Verification items for the finished model (mm, model axes). A direction names the side the tool comes from. Round coordinates to 2 decimals unless told otherwise and drop trailing zeros. Loops run counter-clockwise (first coordinate to the right, second up) from the corner with the lowest first, then second, coordinate; pieces in that order, holes last. Notation, with made-up numbers: M 25,11.5 L 79,11.5 A13 cw 79,19.5 Z; hole C -2.75,68.25 d3. An arc over 180 degrees is marked long. Answer as CSV lines item,"result".
```python
from build123d import *

# Parameters (mm, degrees)
ESQUISSE1_W             = 28
ESQUISSE1_H             = 40
ESQUISSE1_R             = 1.5
BOSS_EXTRU_1_DEPTH      = 1.5
ESQUISSE3_R             = 1.5
ESQUISSE3_W             = 3
ESQUISSE3_H             = 22
BOSS_EXTRU_2_DEPTH      = 1.5
CONG_1_R                = 6
ESQUISSE4_R             = 1.5
ESQUISSE4_W             = 6
ESQUISSE4_H             = 18
ENL_V_MAT_EXTRU_1_DEPTH = 36.387144698
CONG_2_R                = 2


with BuildPart() as part:
    # Esquisse1 → Boss.-Extru.1 (new body)
    with BuildSketch(Plane.XY):
        Rectangle(ESQUISSE1_W, ESQUISSE1_H)
        with Locations((-7.5, 8)):
            Circle(ESQUISSE1_R, mode=Mode.SUBTRACT)
        with Locations(Location((7.5, 8, 0), (0, 0, 180))):
            Circle(ESQUISSE1_R, mode=Mode.SUBTRACT)
        with Locations((7.5, -8)):
            Circle(ESQUISSE1_R, mode=Mode.SUBTRACT)
        with Locations(Location((-7.5, -8, 0), (0, 0, 180))):
            Circle(ESQUISSE1_R, mode=Mode.SUBTRACT)
    extrude(amount=BOSS_EXTRU_1_DEPTH)

    # Esquisse3 → Boss.-Extru.2 (add)
    # profile 1 of 2: a face of its own
    with BuildSketch(Plane.XY.offset(1.5)):
        with BuildLine():
            Line((2, 20), (2, 25))
            ThreePointArc((2, 25), (8, 31), (14, 25))
            Line((14, 25), (14, 20))
            ThreePointArc((14, 20), (8, 14), (2, 20))
        make_face()
        with Locations((8, 25)):
            Circle(ESQUISSE3_R, mode=Mode.SUBTRACT)
    # profile 2 of 2: a face of its own
    with BuildSketch(Plane.XY.offset(1.5)):
        with Locations((-15.5, -9)):
            Rectangle(ESQUISSE3_W, ESQUISSE3_H)
    extrude(amount=-BOSS_EXTRU_2_DEPTH)

    # Congé1
    cong_1_edges = [part.edges().sort_by_distance(p)[0] for p in [
        (2, 20, 0.75),
    ]]
    fillet(cong_1_edges, radius=CONG_1_R)

    # Esquisse4 → Enlèv. mat.-Extru.1 (cut, through all)
    with BuildSketch(Plane.XY.offset(1.5)):
        with Locations((-13.7, -3)):
            Circle(ESQUISSE4_R)
        with Locations(Location((-13.7, -15, 0), (0, 0, 180))):
            Circle(ESQUISSE4_R)
        with Locations((-14, 11)):
            Rectangle(ESQUISSE4_W, ESQUISSE4_H)
    extrude(amount=-ENL_V_MAT_EXTRU_1_DEPTH, mode=Mode.SUBTRACT)

    # Congé2
    cong_2_edges = [part.edges().sort_by_distance(p)[0] for p in [
        (-17, 2, 0.75),
        (-17, -20, 0.75),
        (14, -20, 0.75),
        (-11, 2, 0.75),
        (-11, 20, 0.75),
    ]]
    fillet(cong_2_edges, radius=CONG_2_R)


solid = part.part
```
1) Draft check along Y on faces 3 (the cylindrical face through (13.4, -19.43, 0.76)), 4 (the cylindrical face through (-12.27, -2.55, 0.76)), 5 (the flat face through (2, 0, 1.5)). Enter one of: +Y half, -Y half, draft (parallel to the pull), parting line (faces both ways), or undercut.
Here are the results:
face 3,"-Y half"
face 4,"undercut"
face 5,"draft"
2) Material ranges on probe 1 along Y at (x, z) = (-13.7, 0.6); probe 2 along Y at (x, z) = (8, 0.8); probe 3 along Y at (x, z) = (7.5, 0.45), recorded low to high.
Here are the results:
probe 1,"y = -20 to -16.5, -13.5 to -4.5, -1.5 to 2"
probe 2,"y = -20 to -9.41, -6.59 to 6.59, 9.41 to 23.5, 26.5 to 31"
probe 3,"y = -20 to -9.5, -6.5 to 6.5, 9.5 to 23.59, 26.41 to 30.98"
3) Section check C-C (y = -15). Record the cut outline in (x, z).
Here are the results:
outline,"M -17,0 L -15.2,0 L -15.2,1.5 L -17,1.5 Z; M -12.2,0 L 14,0 L 14,1.5 L -12.2,1.5 Z"
4) Section check A-A (y = 8). Record the cut outline in (x, z).
Here are the results:
outline,"M -11,0 L -9,0 L -9,1.5 L -11,1.5 Z; M -6,0 L 6,0 L 6,1.5 L -6,1.5 Z; M 9,0 L 14,0 L 14,1.5 L 9,1.5 Z"
5) Section check D-D (z = 0.7). State how many separate pieces and enclosed holes the cut face has, plus the area to 3 significant figures.
Here are the results:
separate pieces,"1"
enclosed holes,"7"
area,"1,200 mm^2"
6) Go/stop test with a flat-tipped pin: pin 1 (2.5 mm diameter, centred on x = 7.5, y = -8, fed in from -Z). Record where the tip stops, or that it passes through.
Here are the results:
pin 1,"passes through"
7) Set-up check for faces 1 (the flat face through (-14, 2, 1)), 2 (the cylindrical face through (-16.43, -19.4, 0.74)): record each of +Z, -Z, +X, -X, +Y, -Y from which the full face is reachable in a straight line by a thin tool's end or side.
Here are the results:
face 1,"+Z, -Z, -X, +Y"
face 2,"+Z, -Z, -X, -Y"
8) Section check B-B (x = -7.5). Record the cut outline in (y, z).
Here are the results:
outline,"M -20,0 L -9.5,0 L -9.5,1.5 L -20,1.5 Z; M -6.5,0 L 6.5,0 L 6.5,1.5 L -6.5,1.5 Z; M 9.5,0 L 20,0 L 20,1.5 L 9.5,1.5 Z"
